from build123d import *

# Parameters (mm, degrees)
SKETCH_1_W               = 155
SKETCH_1_H               = 100
EXTRUDE_1_DEPTH          = 5
SKETCH_2_W               = 125
SKETCH_2_H               = 8
EXTRUDE_2_DEPTH          = 25
EXTRUDE_6_DEPTH          = 20
EXTRUDE_7_REACH          = 184.727
EXTRUDE_7_END_RADIUS     = 43.11234224
SKETCH_11_W              = 8
SKETCH_11_H              = 5
SKETCH_12_W              = 125
SKETCH_12_H              = 15
CUT_EXTRUDE_1_DEPTH      = 130
PATTERN_CIRCULAR_1_COUNT = 5
PATTERN_CIRCULAR_1_ANGLE = 90
F_1_THE_OTHER_WAY_COUNT  = 5
F_1_THE_OTHER_WAY_ANGLE  = 90


with BuildPart() as part:
    # 草图1 → 凸台-拉伸1 (new body)
    with BuildSketch(Plane(origin=(0, 0, 0), x_dir=(1, 0, 0), z_dir=(0, 1, 0))):
        with Locations((77.5, 50)):
            Rectangle(SKETCH_1_W, SKETCH_1_H)
    extrude(amount=EXTRUDE_1_DEPTH)

    # 草图2 → 凸台-拉伸2 (add)
    with BuildSketch(Plane(origin=(0, 5, 0), x_dir=(1, 0, 0), z_dir=(0, 1, 0))):
        with Locations((77.5, 4)):
            Rectangle(SKETCH_2_W, SKETCH_2_H)
    extrude(amount=EXTRUDE_2_DEPTH)

    # 草图7 → 凸台-拉伸6 (add)
    with BuildSketch(Plane(origin=(0, 5, 0), x_dir=(1, 0, 0), z_dir=(0, 1, 0))):
        with BuildLine():
            Line((34.50840207, 68.224369845), (40.49159793, 67.775630155))
            ThreePointArc((40.49159793, 67.775630155), (77.5, 27.88765776), (114.50840207, 67.775630155))
            Line((114.50840207, 67.775630155), (120.49159793, 68.224369845))
            ThreePointArc((120.49159793, 68.224369845), (77.5, 21.88765776), (34.50840207, 68.224369845))
        make_face()
    extrude(amount=EXTRUDE_6_DEPTH)

    # 凸台-拉伸7: up to this cylinder (the profile starts outside it)
    extrude_7_end = Plane(origin=(77.5, 22.5, -65), z_dir=(0, -1, 0)) * Cylinder(EXTRUDE_7_END_RADIUS, 456.67868448, mode=Mode.PRIVATE)
    # 草图11 → 凸台-拉伸7 (add, up to the surface)
    with BuildSketch(Plane(origin=(0, 0, -8), x_dir=(-1, 0, 0), z_dir=(0, 0, -1)), mode=Mode.PRIVATE) as extrude_7_sk1:
        with Locations((-77.5, 22.5)):
            Rectangle(SKETCH_11_W, SKETCH_11_H)
    extrude_7_tool1 = extrude(extrude_7_sk1.sketch, amount=EXTRUDE_7_REACH, mode=Mode.PRIVATE) - extrude_7_end
    add(extrude_7_tool1.solids().sort_by_distance((77.5, 22.5, -8))[0])
    # 草图11 → 凸台-拉伸7 (add, up to the surface)
    with BuildSketch(Plane(origin=(0, 0, -8), x_dir=(-1, 0, 0), z_dir=(0, 0, -1)), mode=Mode.PRIVATE) as extrude_7_sk2:
        with Locations((-41.5, 22.5)):
            Rectangle(SKETCH_11_W, SKETCH_11_H)
    extrude_7_tool2 = extrude(extrude_7_sk2.sketch, amount=EXTRUDE_7_REACH, mode=Mode.PRIVATE) - extrude_7_end
    add(extrude_7_tool2.solids().sort_by_distance((41.5, 22.5, -8))[0])
    # 草图11 → 凸台-拉伸7 (add, up to the surface)
    with BuildSketch(Plane(origin=(0, 0, -8), x_dir=(-1, 0, 0), z_dir=(0, 0, -1)), mode=Mode.PRIVATE) as extrude_7_sk3:
        with Locations((-113.5, 22.5)):
            Rectangle(SKETCH_11_W, SKETCH_11_H)
    extrude_7_tool3 = extrude(extrude_7_sk3.sketch, amount=EXTRUDE_7_REACH, mode=Mode.PRIVATE) - extrude_7_end
    add(extrude_7_tool3.solids().sort_by_distance((113.5, 22.5, -8))[0])

    # 草图12 → 切除-拉伸1 (cut)
    with BuildSketch(Plane(origin=(0, 0, -8), x_dir=(-1, 0, 0), z_dir=(0, 0, -1))):
        with Locations((-77.5, 12.5)):
            Rectangle(SKETCH_12_W, SKETCH_12_H)
    extrude(amount=CUT_EXTRUDE_1_DEPTH, mode=Mode.SUBTRACT)

    # 草图16 → 切除-旋转3 (revolve, cut)
    with BuildSketch(Plane(origin=(0, 18, 0), x_dir=(-1, 0, 0), z_dir=(0, -1, 0))):
        with BuildLine():
            Line((-80.5, 25), (-74.5, 25))
            ThreePointArc((-74.5, 25), (-77.5, 22), (-80.5, 25))
        make_face()
    cut_revolve_3 = revolve(axis=Axis((74.5, 18, -25), (1, 0, 0)), mode=Mode.SUBTRACT)

    # 阵列(圆周)1: 切除-旋转3 ×5 about axis
    pattern_circular_1_axis = Axis((77.5, 0, -65), (0, -1, 0))
    for i in range(1, PATTERN_CIRCULAR_1_COUNT):
        add(cut_revolve_3.rotate(pattern_circular_1_axis, i * PATTERN_CIRCULAR_1_ANGLE / (PATTERN_CIRCULAR_1_COUNT - 1)), mode=Mode.SUBTRACT)

    # 1 the other way: 切除-旋转3 ×5 about axis
    f_1_the_other_way_axis = Axis((77.5, 0, -65), (0, 1, 0))
    for i in range(1, F_1_THE_OTHER_WAY_COUNT):
        add(cut_revolve_3.rotate(f_1_the_other_way_axis, i * F_1_THE_OTHER_WAY_ANGLE / (F_1_THE_OTHER_WAY_COUNT - 1)), mode=Mode.SUBTRACT)


solid = part.part
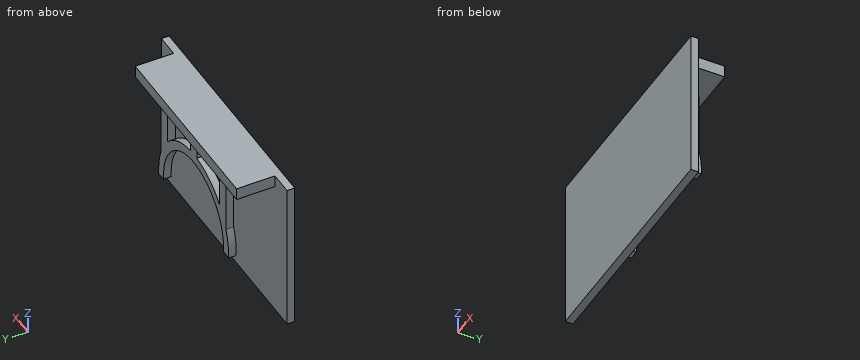
The model under review builds one solid part; all positions refer to its coordinate system, in mm. Round coordinates to 2 decimals unless told otherwise and drop trailing zeros. Order: outer loops, then holes, each group sorted by start corner. A loop starts at its lowest first (then second) coordinate and runs counter-clockwise, first axis right, second up. Notation, with made-up numbers: (54.25, -18.75) -> (79.25, -18.75) arc R30 ccw to (79.25, 3.25) -> close; hole circle Ø4 at (33, 27.5). An arc over 180 degrees is marked (long way). Use CSV: the item, a comma, the result in double quotes. Start each with the question number.
(1) Consider section C-C on y = 10.5. Write out the cut boundary in (x, z).
(2) Insertion check: pin 1 (6 mm diameter, centred on y = 19.5, z = -37, fed in from +X); pin 2 (5.5 mm diameter, centred on y = 23, z = -15.5, fed in from -X); pin 3 (4 mm diameter, centred on x = 19, z = -19.5, fed in from +Y); pin 4 (4 mm diameter, centred on y = 8, z = -88, fed in from +X). Each pin has a flat end and moves straight along its axis. Give the tip position at first contact, or say it passes through.
(3) Wall thickness on probe 1 along Y at (x, z) = (76, -12.5); probe 2 along Y at (x, z) = (144, -45.5); probe 3 along Z at (x, y) = (102, 13.75): over which ranges is each line inside the solid? List them lowest first. Write a range as from..to.
(4) Consider section A-A on z = -65. Write out the cut boundary in (x, y).
(5) Consider section D-D on x = 128. Write out the cut boundary in (y, z), and give its area (3 significant figures).
(6) Consider section B-B on x = 77.5. Write out the cut boundary in (y, z), and give its area (3 significant figures).
Responses:
1,outline,"(15, -8) -> (140, -8) -> (140, 0) -> (15, 0) -> close"
2,pin 1,"x = 117.5"
2,pin 2,"x = 37.5"
2,pin 3,"y = 5"
2,pin 4,"through"
3,probe 1,"0..5, 20..25"
3,probe 2,"0..5"
3,probe 3,"-8..0"
4,outline,"(0, 0) -> (155, 0) -> (155, 5) -> (0, 5) -> close; (34.39, 20) -> (35.26, 20) arc R3 cw to (39.74, 20) -> (40.39, 20) -> (40.39, 25) -> (34.39, 25) -> close; (114.61, 20) -> (115.26, 20) arc R3 cw to (119.74, 20) -> (120.61, 20) -> (120.61, 25) -> (114.61, 25) -> close"
5,outline,"(0, -100) -> (5, -100) -> (5, -8) -> (30, -8) -> (30, 0) -> (0, 0) -> close"
5,area,"700 mm²"
6,outline,"(0, -100) -> (5, -100) -> (5, -8) -> (20, -8) -> (20, -22.76) arc R3 cw to (20, -27.24) -> (20, -27.89) -> (25, -27.89) -> (25, -8) -> (30, -8) -> (30, 0) -> (0, 0) -> close"
6,area,"796 mm²"
